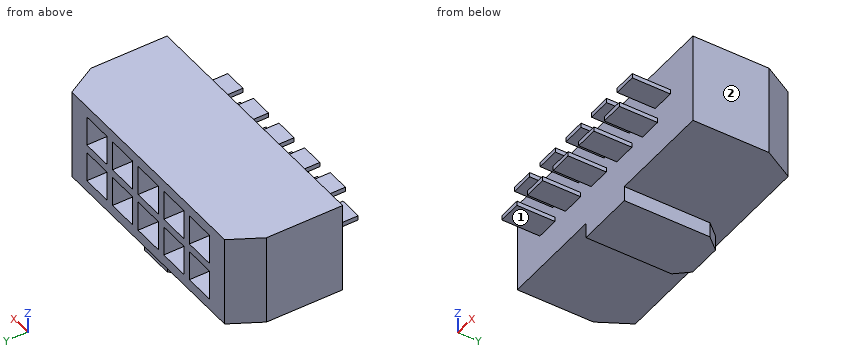
```python
from build123d import *

# Parameters (mm, degrees)
EXTRUDE_1_DEPTH     = 3
EXTRUDE_START       = -4
EXTRUDE_2_DEPTH     = 1
SKETCH_2_W          = 2
SKETCH_2_H          = 2
CUT_EXTRUDE_1_DEPTH = 3
SKETCH_3_W          = 1.5
SKETCH_3_H          = 0.3
EXTRUDE_3_DEPTH     = 2.5


with BuildPart() as part:
    # Эскиз1 → Бобышка-Вытянуть1 (new, symmetric)
    with BuildSketch(Plane.XY):
        Polygon((-8.7, 1.5), (-8.7, -3.5), (-1.9, -3.5), (-1.9, 2.122094745), (-1.129392625, 2.998992793), (1.129392625, 2.998992793), (1.9, 2.122094745), (1.9, -3.5), (8.7, -3.5), (8.7, 1.5), (7.575, 3.5), (-7.575, 3.5), align=None)
        Polygon((-1.9, 2.122094745), (-1.9, -3.5), (1.9, -3.5), (1.9, 2.122094745), (1.129392625, 2.998992793), (-1.129392625, 2.998992793), align=None)
    extrude(amount=EXTRUDE_1_DEPTH, both=True)

    # Эскиз1<3> → Бобышка-Вытянуть2 (add)
    with BuildSketch(Plane.XY.offset(EXTRUDE_START)):
        Polygon((-1.9, 2.122094745), (-1.9, -3.5), (1.9, -3.5), (1.9, 2.122094745), (1.129392625, 2.998992793), (-1.129392625, 2.998992793), align=None)
    extrude(amount=EXTRUDE_2_DEPTH)

    # Эскиз2 → Вырез-Вытянуть1 (cut)
    with BuildSketch(Plane(origin=(0, 3.5, 0), x_dir=(1, 0, 0), z_dir=(0, 1, 0))):
        with Locations((0, 1.27)):
            Rectangle(SKETCH_2_W, SKETCH_2_H)
        with Locations((0, -1.27)):
            Rectangle(SKETCH_2_W, SKETCH_2_H)
        with Locations((2.54, 1.27)):
            Rectangle(SKETCH_2_W, SKETCH_2_H)
        with Locations((2.54, -1.27)):
            Rectangle(SKETCH_2_W, SKETCH_2_H)
        with Locations((-2.54, 1.27)):
            Rectangle(SKETCH_2_W, SKETCH_2_H)
        with Locations((-2.54, -1.27)):
            Rectangle(SKETCH_2_W, SKETCH_2_H)
        with Locations((-5.08, 1.27)):
            Rectangle(SKETCH_2_W, SKETCH_2_H)
        with Locations((-5.08, -1.27)):
            Rectangle(SKETCH_2_W, SKETCH_2_H)
        with Locations((5.08, 1.27)):
            Rectangle(SKETCH_2_W, SKETCH_2_H)
        with Locations((5.08, -1.27)):
            Rectangle(SKETCH_2_W, SKETCH_2_H)
    extrude(amount=-CUT_EXTRUDE_1_DEPTH, mode=Mode.SUBTRACT)

    # Эскиз3 → Бобышка-Вытянуть3 (add)
    with BuildSketch(Plane.XZ.offset(3.5)):
        with Locations((-3.175, -0.575)):
            Rectangle(SKETCH_3_W, SKETCH_3_H)
        with Locations((-1.905, 0.575)):
            Rectangle(SKETCH_3_W, SKETCH_3_H)
        with Locations((-0.635, -0.575)):
            Rectangle(SKETCH_3_W, SKETCH_3_H)
        with Locations((0.635, 0.575)):
            Rectangle(SKETCH_3_W, SKETCH_3_H)
        with Locations((1.905, -0.575)):
            Rectangle(SKETCH_3_W, SKETCH_3_H)
        with Locations((3.175, 0.575)):
            Rectangle(SKETCH_3_W, SKETCH_3_H)
        with Locations((-4.445, 0.575)):
            Rectangle(SKETCH_3_W, SKETCH_3_H)
        with Locations((-5.715, -0.575)):
            Rectangle(SKETCH_3_W, SKETCH_3_H)
        with Locations((5.715, 0.575)):
            Rectangle(SKETCH_3_W, SKETCH_3_H)
        with Locations((4.445, -0.575)):
            Rectangle(SKETCH_3_W, SKETCH_3_H)
    extrude(amount=EXTRUDE_3_DEPTH)


solid = part.part
```
The model under review builds one solid part; all positions refer to its coordinate system, in mm. Face numbers are marked on the shaded views. A direction names the side the tool comes from. Round coordinates to 2 decimals unless told otherwise and drop trailing zeros. Write each loop counter-clockwise with the first axis right and the second up, starting at its lowest first coordinate (ties: lowest second). Pieces come first, ordered by that corner, then holes. Notation, with made-up numbers: M -30.5,-3.5 L -18.5,-3.5 A12 ccw -18.5,2.5 Z; hole C 49.25,-24 d6. An arc over 180 degrees is marked long. Use CSV: the item, a comma, the result in double quotes. Start each with the question number.
(1) We need section A-A, the plane x = -4.5. State the section outline as (y, z) points (3 decimals), then the cut area to 4 significant figures.
(2) We need section C-C, the plane y = 0.75. State how many separate pieces and enclosed holes the cut face has, then the cut area to 3 significant figures.
(3) We need section D-D, the plane y = -3.25. State the section outline as (x, z) points.
(4) Clearance check with flat-ended pins moving along their axes: P1, Ø1.6, axis at x = -3, y = -4.5, coming from the -Z side (3 decimals); P2, Ø1, axis at x = -2.5, y = 2, coming from the -Z side; P3, Ø0.5, axis at x = -2, y = -4.5, coming from the -Z side (3 decimals). State where each tip first meets the part, or that it passes through.
(5) For line 1 along Z through (x, y) = (5, 2.5); line 2 along X through (y, z) = (-4.75, -0.5) (3 decimals); line 3 along X through (y, z) = (1.5, -1.5), list the stretches that pass through material, from the lowest coordinate up.
(6) Tool access review of the marked faces 1 and 2: name each direction out of +Z, -Z, +X, -X, +Y, -Y from which nothing blocks a thin tool from reaching the whole face with its end or side.
(7) We need section B-B, the plane z = -2. State the section outline as (x, y) points (3 decimals).
Findings:
1,outline,"M -6,0.425 L -3.5,0.425 L -3.5,-3 L 3.5,-3 L 3.5,-2.27 L 0.5,-2.27 L 0.5,-0.27 L 3.5,-0.27 L 3.5,0.27 L 0.5,0.27 L 0.5,2.27 L 3.5,2.27 L 3.5,3 L -3.5,3 L -3.5,0.725 L -6,0.725 Z"
1,area,"30.75 mm^2"
2,separate pieces,"1"
2,enclosed holes,"10"
2,area,"68.2 mm^2"
3,outline,"M -8.7,-3 L -1.9,-3 L -1.9,-4 L 1.9,-4 L 1.9,-3 L 8.7,-3 L 8.7,3 L -8.7,3 Z"
4,P1,"z = -0.725"
4,P2,"z = -3"
4,P3,"z = 0.425"
5,line 1,"-3 to -2.27, -0.27 to 0.27, 2.27 to 3"
5,line 2,"-6.465 to -4.965, -3.925 to -2.425, -1.385 to 0.115, 1.155 to 2.655, 3.695 to 5.195"
5,line 3,"-8.7 to -6.08, -4.08 to -3.54, -1.54 to -1, 1 to 1.54, 3.54 to 4.08, 6.08 to 8.7"
6,face 1,"-Z, +X, -X, -Y"
6,face 2,"+Z, -Z, +X, +Y, -Y"
7,outline,"M -8.7,-3.5 L 8.7,-3.5 L 8.7,1.5 L 7.575,3.5 L 6.08,3.5 L 6.08,0.5 L 4.08,0.5 L 4.08,3.5 L 3.54,3.5 L 3.54,0.5 L 1.54,0.5 L 1.54,3.5 L 1,3.5 L 1,0.5 L -1,0.5 L -1,3.5 L -1.54,3.5 L -1.54,0.5 L -3.54,0.5 L -3.54,3.5 L -4.08,3.5 L -4.08,0.5 L -6.08,0.5 L -6.08,3.5 L -7.575,3.5 L -8.7,1.5 Z"
